Can you work these out from the model? Positions are in its coordinate system, mm. A direction names the side the tool comes from. Give positions to 0.01 mm unless a question says otherwise; leave off trailing zeros. Write each loop counter-clockwise with the first axis right and the second up, starting at its lowest first coordinate (ties: lowest second). Pieces come first, ordered by that corner, then holes.
```python
from build123d import *

# Parameters (mm, degrees)
CROQUIS1_R              = 7
SALIENTE_EXTRUIR1_DEPTH = 2
CROQUIS2_R              = 6
CROQUIS2_R_2            = 4.25
SALIENTE_EXTRUIR2_DEPTH = 6
REDONDEO3_R             = 2
REDONDEO4_R             = 1
CROQUIS3_R              = 3.75
CROQUIS3_R_2            = 3.25
SALIENTE_EXTRUIR3_DEPTH = 3


with BuildPart() as part:
    # Croquis1 → Saliente-Extruir1 (new body)
    with BuildSketch(Plane(origin=(0, 0, 0), x_dir=(1, 0, 0), z_dir=(0, 1, 0))):
        with Locations(Location((0, 0, 0), (0, 0, 270))):
            Circle(CROQUIS1_R)
    extrude(amount=SALIENTE_EXTRUIR1_DEPTH)

    # Croquis2 → Saliente-Extruir2 (add)
    with BuildSketch(Plane(origin=(0, 2, 0), x_dir=(1, 0, 0), z_dir=(0, 1, 0))):
        with Locations(Location((0, 0, 0), (0, 0, 270))):
            Circle(CROQUIS2_R)
        with Locations(Location((0, 0, 0), (0, 0, 270))):
            Circle(CROQUIS2_R_2, mode=Mode.SUBTRACT)
    extrude(amount=SALIENTE_EXTRUIR2_DEPTH)

    # Redondeo3
    redondeo3_edges = [part.edges().sort_by_distance(p)[0] for p in [
        (0, 2, -4.25),
    ]]
    fillet(redondeo3_edges, radius=REDONDEO3_R)

    # Redondeo4
    redondeo4_edges = [part.edges().sort_by_distance(p)[0] for p in [
        (0, 2, -6),
    ]]
    fillet(redondeo4_edges, radius=REDONDEO4_R - 0.0001)  # a hair under: the kernel refuses the full size

    # Croquis3 → Saliente-Extruir3 (add)
    with BuildSketch(Plane.XZ):
        with Locations(Location((0, 0, 0), (0, 0, 90))):
            Circle(CROQUIS3_R)
        with Locations(Location((0, 0, 0), (0, 0, 270))):
            Circle(CROQUIS3_R_2, mode=Mode.SUBTRACT)
    extrude(amount=SALIENTE_EXTRUIR3_DEPTH)


solid = part.part
```
1) Please list where these lines run through material, in increasing order: L1, parallel to X at y = 5.6, z = 0; L2, parallel to X at y = -2.35, z = 0; L3, parallel to Y at x = -2.75, z = -4.
Values follow:
L1: x = -6 to -4.25, 4.25 to 6
L2: x = -3.75 to -3.25, 3.25 to 3.75
L3: y = 0 to 8
2) Suppose I cut it at A-A on y = 4.5. Write out the boundary of the cut face in (x, z), plus the area to 3 significant figures.
Values follow:
outline: circle Ø12 at (0, 0); hole circle Ø8.5 at (0, 0)
area: 56.4 mm2
3) Suppose I cut it at D-D on y = -0.25. Write out the boundary of the cut face in (x, z).
Values follow:
outline: circle Ø7.5 at (0, 0); hole circle Ø6.5 at (0, 0)
4) For faces 4 (the face through (1.802, 5.465, 5.723)), 5 (the face through (-3.1, -3, -1.4)), 6 (the face through (0, 0, 0)), which set-ups out of +Z, -Z, +X, -X, +Y, -Y let a thin tool reach every point of the face, with its end or its side?
Values follow:
face 4: +Y
face 5: +Z, -Z, +X, -X, -Y
face 6: -Y
5) If we mould it in two halves opening along X, with no side actions, what happens to faces 1 (the face through (-1.978, -1.479, 2.579)), 2 (the face through (-0.165, -1.479, -3.746)), 3 (the face through (-3, 0, 3))? For each: +X half, -X half, draft (parallel to the pull), parting line (faces both ways), or undercut.
Values follow:
face 1: undercut
face 2: parting line
face 3: draft
6) For pin 1 Ø6 at (x, y) = (5, 4.5) entering from -Z; pin 2 Ø3.5 at (x, z) = (0, 0) entering from +Y; pin 3 Ø1.5 at (y, z) = (1.5, -2.5) entering from -X, each with a flat end and sliding along its axis, tell me the tip position at first contact or that it passes through.
Values follow:
pin 1: stops at z = -6.15
pin 2: stops at y = 2
pin 3: stops at x = -6.78
